```python
from build123d import *

# Parameters (mm, degrees)
PAD096_DEPTH                       = 3
SKETCH195_R                        = 1.5
POCKET075_DEPTH                    = 5
POLARPATTERN011_COUNT              = 4
SKETCH196_R                        = 1.5
POCKET076_DEPTH                    = 5
SKETCH196_LINEARPATTERN003_2_R     = 1.5
POCKET076_LINEARPATTERN003_2_DEPTH = 5
SKETCH196_LINEARPATTERN003_3_R     = 1.5
POCKET076_LINEARPATTERN003_3_DEPTH = 5
SKETCH196_LINEARPATTERN003_4_R     = 1.5
POCKET076_LINEARPATTERN003_4_DEPTH = 5
SKETCH196_LINEARPATTERN003_5_R     = 1.5
POCKET076_LINEARPATTERN003_5_DEPTH = 5
LINEARPATTERN004_COUNT             = 3
LINEARPATTERN004_PITCH             = 10
SKETCH197_R                        = 1.5
POCKET077_DEPTH                    = 5
SKETCH206_R                        = 1.5
POCKET081_DEPTH                    = 311.766283
SKETCH206_MIRRORED001_2_R          = 1.5
POCKET081_MIRRORED001_2_DEPTH      = 311.766283
SKETCH207_R                        = 1.5
POCKET082_DEPTH                    = 5
SKETCH207_MIRRORED003_2_R          = 1.5
POCKET082_MIRRORED003_2_DEPTH      = 5
SKETCH220_R                        = 1.5
POCKET089_DEPTH                    = 5
BODY074_ROLL_ANGLE                 = 90
BODY074_PLACEMENT_ANGLE            = 90


with BuildPart() as part:
    # Sketch194 → Pad096 (new body)
    with BuildSketch(Plane(origin=(0, 0, 0), x_dir=(-1, 0, 0), z_dir=(0, 1, 0))):
        with BuildLine():
            Line((-60, 30), (60, 30))
            ThreePointArc((70, 20), (67.071068, 27.071068), (60, 30))
            Line((70, 20), (70, -25))
            ThreePointArc((60, -35), (67.071068, -32.071068), (70, -25))
            Line((60, -35), (-60, -35))
            ThreePointArc((-70, -25), (-67.071068, -32.071068), (-60, -35))
            Line((-70, 20), (-70, -25))
            ThreePointArc((-60, 30), (-67.071068, 27.071068), (-70, 20))
        make_face()
    extrude(amount=PAD096_DEPTH)

    # Sketch195 (on Face10 of Pad096) → Pocket075 (cut)
    with BuildSketch(Plane(origin=(0, 3, 0), x_dir=(1, 0, 0), z_dir=(0, 1, 0))):
        with Locations((10, -10)):
            Circle(SKETCH195_R)
    pocket075 = extrude(amount=-POCKET075_DEPTH, mode=Mode.SUBTRACT)

    # PolarPattern011: Pocket075 ×4 about axis
    polarpattern011_axis = Axis((0, 3, 0), (0, 1, 0))
    for i in range(1, POLARPATTERN011_COUNT):
        add(pocket075.rotate(polarpattern011_axis, i * 360 / POLARPATTERN011_COUNT), mode=Mode.SUBTRACT)

    # Sketch196 (on Face5 of PolarPattern011) → Pocket076 (cut)
    with BuildSketch(Plane(origin=(65, 3, -5), x_dir=(1, 0, 0), z_dir=(0, 1, 0))):
        Circle(SKETCH196_R)
    pocket076 = extrude(amount=-POCKET076_DEPTH, mode=Mode.SUBTRACT)

    # Sketch196 LinearPattern003 2 → Pocket076 LinearPattern003 2 (cut)
    with BuildSketch(Plane(origin=(55, 3, -5), x_dir=(1, 0, 0), z_dir=(0, 1, 0))):
        Circle(SKETCH196_LINEARPATTERN003_2_R)
    pocket076_linearpattern003_2 = extrude(amount=-POCKET076_LINEARPATTERN003_2_DEPTH, mode=Mode.SUBTRACT)

    # Sketch196 LinearPattern003 3 → Pocket076 LinearPattern003 3 (cut)
    with BuildSketch(Plane(origin=(45, 3, -5), x_dir=(1, 0, 0), z_dir=(0, 1, 0))):
        Circle(SKETCH196_LINEARPATTERN003_3_R)
    pocket076_linearpattern003_3 = extrude(amount=-POCKET076_LINEARPATTERN003_3_DEPTH, mode=Mode.SUBTRACT)

    # Sketch196 LinearPattern003 4 → Pocket076 LinearPattern003 4 (cut)
    with BuildSketch(Plane(origin=(35, 3, -5), x_dir=(1, 0, 0), z_dir=(0, 1, 0))):
        Circle(SKETCH196_LINEARPATTERN003_4_R)
    pocket076_linearpattern003_4 = extrude(amount=-POCKET076_LINEARPATTERN003_4_DEPTH, mode=Mode.SUBTRACT)

    # Sketch196 LinearPattern003 5 → Pocket076 LinearPattern003 5 (cut)
    with BuildSketch(Plane(origin=(25, 3, -5), x_dir=(1, 0, 0), z_dir=(0, 1, 0))):
        Circle(SKETCH196_LINEARPATTERN003_5_R)
    pocket076_linearpattern003_5 = extrude(amount=-POCKET076_LINEARPATTERN003_5_DEPTH, mode=Mode.SUBTRACT)

    # LinearPattern004: Pocket076, Pocket076 LinearPattern003 2, Pocket076 LinearPattern003 3, Pocket076 LinearPattern003 4, Pocket076 LinearPattern003 5 ×3
    with Locations(*[(0, 0, -i * LINEARPATTERN004_PITCH) for i in range(1, LINEARPATTERN004_COUNT)]):
        add(pocket076, mode=Mode.SUBTRACT)
        add(pocket076_linearpattern003_2, mode=Mode.SUBTRACT)
        add(pocket076_linearpattern003_3, mode=Mode.SUBTRACT)
        add(pocket076_linearpattern003_4, mode=Mode.SUBTRACT)
        add(pocket076_linearpattern003_5, mode=Mode.SUBTRACT)

    # Sketch197 (on Face5 of MultiTransform) → Pocket077 (cut)
    with BuildSketch(Plane(origin=(0, 3, 0), x_dir=(1, 0, 0), z_dir=(0, 1, 0))):
        with Locations((-66, -9)):
            Circle(SKETCH197_R)
        with Locations((-66, -19)):
            Circle(SKETCH197_R)
        with Locations((-15.5, -9)):
            Circle(SKETCH197_R)
        with Locations((-15.5, -19)):
            Circle(SKETCH197_R)
        with BuildLine():
            Line((-19.25, -24), (-19.25, -4))
            ThreePointArc((-20.25, -3), (-19.542893, -3.292893), (-19.25, -4))
            Line((-20.25, -3), (-61.25, -3))
            ThreePointArc((-62.25, -4), (-61.957107, -3.292893), (-61.25, -3))
            Line((-62.25, -4), (-62.25, -24))
            ThreePointArc((-61.25, -25), (-61.957107, -24.707107), (-62.25, -24))
            Line((-61.25, -25), (-20.25, -25))
            ThreePointArc((-19.25, -24), (-19.542893, -24.707107), (-20.25, -25))
        make_face()
    extrude(amount=-POCKET077_DEPTH, mode=Mode.SUBTRACT)

    # Sketch206 → Pocket081 (cut, through all)
    with BuildSketch(Plane(origin=(50, 0, 11.5), x_dir=(1, 0, 0), z_dir=(0, -1, 0))):
        with Locations((15, 4)):
            Circle(SKETCH206_R)
    pocket081 = extrude(amount=-POCKET081_DEPTH, mode=Mode.SUBTRACT)

    # Sketch206 Mirrored001 2 → Pocket081 Mirrored001 2 (cut, through all)
    with BuildSketch(Plane(origin=(50, 0, 11.5), x_dir=(-1, 0, 0), z_dir=(0, 1, 0))):
        with Locations((15, 4)):
            Circle(SKETCH206_MIRRORED001_2_R)
    pocket081_mirrored001_2 = extrude(amount=POCKET081_MIRRORED001_2_DEPTH, mode=Mode.SUBTRACT)

    # Mirrored002: Pocket081, Pocket081 Mirrored001 2 across Sketch206 H_Axis
    add(pocket081.mirror(Plane(origin=(50, 0, 11.5), x_dir=(0, -1, 0), z_dir=(0, 0, 1))), mode=Mode.SUBTRACT)
    add(pocket081_mirrored001_2.mirror(Plane(origin=(50, 0, 11.5), x_dir=(0, -1, 0), z_dir=(0, 0, 1))), mode=Mode.SUBTRACT)

    # Sketch207 → Pocket082 (cut)
    with BuildSketch(Plane(origin=(-50, 0, -13.5), x_dir=(1, 0, 0), z_dir=(0, -1, 0))):
        with Locations((15, 4)):
            Circle(SKETCH207_R)
    pocket082 = extrude(amount=-POCKET082_DEPTH, mode=Mode.SUBTRACT)

    # Sketch207 Mirrored003 2 → Pocket082 Mirrored003 2 (cut)
    with BuildSketch(Plane(origin=(-50, 0, -13.5), x_dir=(-1, 0, 0), z_dir=(0, 1, 0))):
        with Locations((15, 4)):
            Circle(SKETCH207_MIRRORED003_2_R)
    pocket082_mirrored003_2 = extrude(amount=POCKET082_MIRRORED003_2_DEPTH, mode=Mode.SUBTRACT)

    # Mirrored004: Pocket082, Pocket082 Mirrored003 2 across Sketch207 H_Axis
    add(pocket082.mirror(Plane(origin=(-50, 0, -13.5), x_dir=(0, -1, 0), z_dir=(0, 0, 1))), mode=Mode.SUBTRACT)
    add(pocket082_mirrored003_2.mirror(Plane(origin=(-50, 0, -13.5), x_dir=(0, -1, 0), z_dir=(0, 0, 1))), mode=Mode.SUBTRACT)

    # Sketch220 → Pocket089 (cut)
    with BuildSketch(Plane(origin=(18, 0, 0), x_dir=(1, 0, 0), z_dir=(0, -1, 0))):
        with Locations((0, 9)):
            Circle(SKETCH220_R)
        with Locations((0, -9)):
            Circle(SKETCH220_R)
    extrude(amount=-POCKET089_DEPTH, mode=Mode.SUBTRACT)


with BuildPart() as part_1:
    # Body074 roll: moved
    add(part.part.rotate(Axis((0, 0, 0), (1, 0, 0)), BODY074_ROLL_ANGLE))


with BuildPart() as part_2:
    # Body074 placement: moved
    add(part_1.part.moved(Location((25, 0, 13))).rotate(Axis((25, 0, 13), (0, 0, 1)), BODY074_PLACEMENT_ANGLE))


solid = part_2.part
```
Part model, mm, in its own coordinate system. Round coordinates to 2 decimals unless told otherwise and drop trailing zeros. Loops run counter-clockwise (first coordinate to the right, second up) from the corner with the lowest first, then second, coordinate; pieces in that order, holes last.
1. Drill centre lines: line 1 along X through (y, z) = (-10, 14.55); line 2 along X through (y, z) = (18, 14.7); line 3 along X through (y, z) = (-37, 13.6). Where is each one in solid material? Low to high.
Solutions:
line 1: x = -10 to 13.5, 16.5 to 33.5, 36.5 to 55
line 2: x = -10 to 14.5, 17.5 to 32.5, 35.5 to 55
line 3: x = -10 to 28, 50 to 55
2. Slice it at C-C (x = 20). Give the cut face in (y, z).
Solutions:
outline: (-70, 13) - (23.5, 13) - (23.5, 16) - (-70, 16) - close; (26.5, 13) - (33.5, 13) - (33.5, 16) - (26.5, 16) - close; (36.5, 13) - (43.5, 13) - (43.5, 16) - (36.5, 16) - close; (46.5, 13) - (53.5, 13) - (53.5, 16) - (46.5, 16) - close; (56.5, 13) - (63.5, 13) - (63.5, 16) - (56.5, 16) - close; (66.5, 13) - (70, 13) - (70, 16) - (66.5, 16) - close
3. Slice it at A-A (x = 40.5). Give the cut face in (y, z), and give its area (3 significant figures).
Solutions:
outline: (-70, 13) - (-62.25, 13) - (-62.25, 16) - (-70, 16) - close; (-19.25, 13) - (33.5, 13) - (33.5, 16) - (-19.25, 16) - close; (36.5, 13) - (63.5, 13) - (63.5, 16) - (36.5, 16) - close; (66.5, 13) - (70, 13) - (70, 16) - (66.5, 16) - close
area: 273 mm2
4. Slice it at B-B (y = -54.5). Give the cut face in (x, z), and give its area (3 significant figures).
Solutions:
outline: (-10, 13) - (28, 13) - (28, 16) - (-10, 16) - close; (50, 13) - (55, 13) - (55, 16) - (50, 16) - close
area: 129 mm2
5. Flat gauge pin, fed straight in: pin 1 (2.5 mm diameter, centred on x = 16, y = 18, fed in from +Z). Where does the tip first touch, or does it go through?
Solutions:
pin 1: passes through
6. Two-plate mould, pull along X, no slides. Class faces 1 (the face through (-7.15, -66.99, 14.48)), 2 (the face through (23, 70, 14)), 3 (the face through (34.575, -64.614, 14.521)): pulls with the +X half, pulls with the -X half, needs draft (parallel to the pull), parting line crosses it, or undercut.
Solutions:
face 1: pulls with the -X half
face 2: needs draft
face 3: undercut
7. Slice it at D-D (y = 25). Give the cut face in (x, z).
Solutions:
outline: (-10, 13) - (-1.5, 13) - (-1.5, 16) - (-10, 16) - close; (1.5, 13) - (8.5, 13) - (8.5, 16) - (1.5, 16) - close; (11.5, 13) - (18.5, 13) - (18.5, 16) - (11.5, 16) - close; (21.5, 13) - (55, 13) - (55, 16) - (21.5, 16) - close
